Autodesk Inventor part; units mm, degrees
ref_plane "Work Plane1" through (0, -6, 0) normal (1, 0, 0) x (0, 0, 1)
ref_plane "YZ Plane" through (0, 0, 0) normal (1, 0, 0) x (0, 1, 0)
ref_plane "XZ Plane" through (0, 0, 0) normal (0, 1, 0) x (-1, 0, 0)
sketch "Náčrt1" plane through (0, 0, 0) normal (0, 0, 1) x (1, 0, 0)
  line L0 (-6, 0) -> (6, 0) construction
  arc A0 (0.425, -11.7343) -> (-0.425, -11.7343) centre (0, -6) ccw
  line L1 (0, 20.1894) -> (0, -80.5364)
  line L2 (-48.09, 0) -> (48.09, 0)
  line L3 (-0.425, -11.7343) -> (-0.425, -14.9343)
  line L4 (-0.425, -6.5402) -> (-0.425, -13.29) construction
  line L5 (-2.7947, 2) -> (3.6722, 2) construction
  arc A1 (4.156, -11.7432) -> (-4.156, -11.7432) centre (0, -5.5) ccw
  arc A2 (-2.0989, -14.6946) -> (-0.425, -14.9343) centre (0, -6) ccw
  arc A3 (-3.399, -13.1002) -> (-2.0989, -14.6946) centre (-1.7, -13.0421) ccw
  arc A4 (-3.399, -13.1002) -> (-4.156, -11.7432) centre (-5.098, -13.1583) ccw
  line L6 (0.425, -11.7343) -> (0.425, -14.9343)
  line L7 (0.425, -6.5402) -> (0.425, -13.29) construction
  arc A5 (0.425, -14.9343) -> (2.0989, -14.6946) centre (0, -6) ccw
  arc A6 (2.0989, -14.6946) -> (3.399, -13.1002) centre (1.7, -13.0421) ccw
  arc A7 (4.156, -11.7432) -> (3.399, -13.1002) centre (5.098, -13.1583) ccw
  circle A8 centre (-1.7, -13.0421) radius 0.85
  circle A9 centre (1.7, -13.0421) radius 0.85
  dimension "d0" = 11.5
  dimension "d1" = 3.2
  dimension "d6" = 0.425
  dimension "d7" = 2
  dimension "d8" = 0.5
  dimension "d9" = 1.7
  dimension "d10" = 1.7
  dimension "d11" = 1.275
  dimension "d12" = 1.7
  dimension "d13" = 1.7
  dimension "d14" = 6
extrude "Těleso" add sketch "Náčrt1" along normal blind 1
ref_plane "Work Plane1" through (0, -6, 0) normal (1, 0, 0) x (0, 0, 1)
equation "\"d0\" = ND"
equation "\"d1\" = SRB2"
equation "\"d6\" = 0.25 * SD5"
equation "\"d7\" = SRB1"
equation "\"d8\" = 0.25 * SRB1"
equation "\"d9\" = SD5"
equation "\"d10\" = SD5"
equation "\"d11\" = 0.75 * SD5"
equation "\"d12\" = SD5"
equation "\"d13\" = SD5"
equation "\"d14\" = 0.5 * WD"
equation "\"d2\" = SD"
equation "\"WD\" = WDMIN"
equation "\"SD\" = 1"
equation "\"SRB1\" = 2"
equation "\"ND\" = 11.5"
equation "\"SRB2\" = 3.2"
equation "\"SD5\" = 1.7"
equation "\"WDMIN\" = 12"
equation "\"SD3\" = 11"
equation "\"WDMAX\" = 13"
properties part number "CSN 02 2930 - 12" material "Nerezová ocel"
Can you work these out from the model? Positions are in its coordinate system, mm. A direction names the side the tool comes from. Coordinates: 2 decimals unless noted, no trailing zeros. Write each loop counter-clockwise with the first axis right and the second up, starting at its lowest first coordinate (ties: lowest second). Pieces come first, ordered by that corner, then holes. Notation, with made-up numbers: (62.5, 70.25) -> (120.5, 70.25) arc R19 ccw to (120.5, 95.25) -> close; hole circle Ø9 at (29, 54). An arc over 180 degrees is marked (long way). Write each question's results on one line, items separated by ' | '. Start each with the question number.
Q1. Imagine slicing it at C-C (z = 0.7). Write out the boundary of the cut face in (x, y) (3 decimals).
Q2. If I drill on probe 1 along Y at (x, z) = (1.7, 0.3); probe 2 along Y at (x, z) = (-2, 0.15); probe 3 along X at (y, z) = (-4.75, 0.65), over which ranges is the centre line in solid material (lowest first)?
Q3. Imagine slicing it at B-B (x = -1.7). Write out the boundary of the cut face in (y, z), then the cut area to 3 significant figures.
Q4. Imagine slicing it at D-D (x = -5.5). Write out the boundary of the cut face in (y, z).
Q5. Imagine slicing it at A-A (y = -6.5). Write out the boundary of the cut face in (x, z).
Q6. We'd pull the mould along X, two halves only. Please class faces 3 (the face through (-3.008, -14.128, 0.493)), 4 (the face through (1.589, -13.885, 0.493)), 5 (the face through (3.03, -14.1, 0.49)): +X half, -X half, draft (parallel to the pull), parting line (faces both ways), or undercut.
Q7. I'm going to push a flat-ended pin straight in: pin 1 (0.5 mm diameter, centred on y = -13, z = 0.5, fed in from -X). Where does the tip first touch, or does it pass through?
Q8. On a 3-axis mill with a long thin cutter (end or side, diameter ignored), from which of +Z, -Z, +X, -X, +Y, -Y can I reach the whole of each face in a straight line? I mean faces 1 (the face through (0.425, -13.3, 0.5)), 2 (the face through (0, 0, 1)). Say none if no direction works.
Taken from the geometry:
1) outline: (-4.156, -11.743) arc R1.7 cw to (-3.399, -13.1) arc R1.7 ccw to (-2.099, -14.695) arc R8.95 ccw to (-0.425, -14.934) -> (-0.425, -11.734) arc R5.75 cw (long way) to (0.425, -11.734) -> (0.425, -14.934) arc R8.939 ccw to (2.099, -14.695) arc R1.7 ccw to (3.399, -13.1) arc R1.7 cw to (4.156, -11.743) arc R7.5 ccw (long way) to start; hole circle Ø1.7 at (-1.7, -13.042); hole circle Ø1.7 at (1.7, -13.042)
2) probe 1: y = -14.78 to -13.89, -12.19 to -11.49, -0.51 to 1.8 | probe 2: y = -14.72 to -13.84, -12.25 to -11.39, -0.61 to 1.73 | probe 3: x = -7.46 to -5.61, 5.61 to 7.46
3) outline: (-14.78, 0) -> (-13.89, 0) -> (-13.89, 1) -> (-14.78, 1) -> close; (-12.19, 0) -> (-11.49, 0) -> (-11.49, 1) -> (-12.19, 1) -> close; (-0.51, 0) -> (1.8, 0) -> (1.8, 1) -> (-0.51, 1) -> close | area: 3.90 mm^2
4) outline: (-10.6, 0) -> (-7.68, 0) -> (-7.68, 1) -> (-10.6, 1) -> close; (-4.32, 0) -> (-0.4, 0) -> (-0.4, 1) -> (-4.32, 1) -> close
5) outline: (-7.43, 0) -> (-5.73, 0) -> (-5.73, 1) -> (-7.43, 1) -> close; (5.73, 0) -> (7.43, 0) -> (7.43, 1) -> (5.73, 1) -> close
6) face 3: -X half | face 4: undercut | face 5: +X half
7) pin 1: stops at x = -3.45
8) face 1: +Z, -Z, -Y | face 2: +Z, +X, -X, +Y, -Y
